Verification items for the finished model (mm, model axes). Face numbers are marked on the shaded views. A direction names the side the tool comes from. Round coordinates to 2 decimals unless told otherwise and drop trailing zeros. Write each loop counter-clockwise with the first axis right and the second up, starting at its lowest first coordinate (ties: lowest second). Pieces come first, ordered by that corner, then holes. Notation, with made-up numbers: M -37.5,61 L 3.5,61 A36 cw 3.5,97 Z; hole C 73.5,50 d11. An arc over 180 degrees is marked long. One line per item, written item: value. Start each with the question number.
Item 1: Section check D-D, the plane z = -10. Record the cut outline in (x, y), then the cut area to 3 significant figures.
Item 2: Gauge pin test, flat ends, axial feed: pin 1 (5.5 mm diameter, centred on x = 26, y = 11.5, fed in from +Z); pin 2 (12 mm diameter, centred on x = -13, y = 17, fed in from -Z); pin 3 (4 mm diameter, centred on x = 55.97, z = 20.76, fed in from +Y); pin 4 (3 mm diameter, centred on y = 13.5, z = 16, fed in from -X). Record the tip position at first contact, or that the pin passes through.
Item 3: Thickness scan on probe 1 along X at (y, z) = (31.5, -2); probe 2 along Y at (x, z) = (48.5, -8); probe 3 along Y at (x, z) = (-3, -3). Record the ranges inside material, lowest first. Write a range as from..to.
Item 4: Tool access check on the marked faces 5, 6, 7 and 8. Record the directions out of +Z, -Z, +X, -X, +Y, -Y that give a thin tool (end or side, any length) a straight path to the whole face; none if there is none.
Item 5: Draft check along X on the marked faces 1, 2, 3 and 4. Enter one of: +X half, -X half, draft (parallel to the pull), parting line (faces both ways), or undercut.
Item 6: Section check B-B, the plane y = 7. Record the cut outline in (x, z).
Item 7: Section check A-A, the plane y = 12.5. Record the cut outline in (x, z), then the cut area to 3 significant figures.
Item 8: Section check C-C, the plane x = 39.5. Record the cut outline in (y, z).
from build123d import *

# Parameters (mm, degrees)
CROQUIS1_W              = 98
CROQUIS1_H              = 53
SALIENTE_EXTRUIR1_DEPTH = 35
CROQUIS2_R              = 1.052356083
CORTAR_EXTRUIR1_DEPTH   = 25
CROQUIS4_R              = 1.21
CORTAR_EXTRUIR2_DEPTH   = 77.456439381
CROQUIS5_R              = 1.21
CORTAR_EXTRUIR3_DEPTH   = 77.456439381
CROQUIS6_W              = 19.087146806
CROQUIS6_H              = 12.5
CORTAR_EXTRUIR4_DEPTH   = 99.715019882
CROQUIS7_W              = 19.109936399
CROQUIS7_H              = 12.5
CORTAR_EXTRUIR5_DEPTH   = 95.352926478
CORTAR_EXTRUIR6_DEPTH   = 83.575081806
CORTAR_EXTRUIR7_DEPTH   = 30
CORTAR_EXTRUIR8_DEPTH   = 110.416374403
CORTAR_EXTRUIR9_DEPTH   = 24
CROQUIS12_W             = 107.668440241
CROQUIS12_H             = 57.968086936
CORTAR_EXTRUIR10_DEPTH  = 2.5
CORTAR_EXTRUIR11_DEPTH  = 109.642500834


with BuildPart() as part:
    # Croquis1 → Saliente-Extruir1 (new body)
    with BuildSketch(Plane(origin=(0, 0, 0), x_dir=(1, 0, 0), z_dir=(0, 1, 0))):
        with Locations((9.971553611, -7.307439825)):
            Rectangle(CROQUIS1_W, CROQUIS1_H)
    extrude(amount=SALIENTE_EXTRUIR1_DEPTH)

    # Croquis2 → Cortar-Extruir1 (cut)
    with BuildSketch(Plane(origin=(0, 35, 0), x_dir=(1, 0, 0), z_dir=(0, 1, 0))):
        Polygon((19.971553611, -26.807439825), (9.971553611, -26.807439825), (-0.028446389, -26.807439825), (-21.028702453, -26.807439825), (-36.028446389, -15.003760101), (-39.028446389, -12.284028263), (-39.028446389, -33.807439825), (58.971553611, -33.807439825), (58.971553611, -10.155599963), (55.971553611, -15.003760101), (40.942820659, -26.807439825), align=None)
        with Locations(Location((-36.028446389, -20.755083742, 0), (0, 0, 270))):
            Circle(CROQUIS2_R, mode=Mode.SUBTRACT)
        with Locations(Location((55.971553611, -20.755083742, 0), (0, 0, 270))):
            Circle(CROQUIS2_R, mode=Mode.SUBTRACT)
    extrude(amount=-CORTAR_EXTRUIR1_DEPTH, mode=Mode.SUBTRACT)

    # Croquis4 → Cortar-Extruir2 (cut, through all)
    with BuildSketch(Plane(origin=(0, 35, 0), x_dir=(1, 0, 0), z_dir=(0, 1, 0))):
        with Locations(Location((-36.028446389, -20.755083742, 0), (0, 0, 270))):
            Circle(CROQUIS4_R)
    extrude(amount=-CORTAR_EXTRUIR2_DEPTH, mode=Mode.SUBTRACT)

    # Croquis5 → Cortar-Extruir3 (cut, through all)
    with BuildSketch(Plane(origin=(0, 35, 0), x_dir=(1, 0, 0), z_dir=(0, 1, 0))):
        with Locations(Location((55.971553611, -20.755083742, 0), (0, 0, 270))):
            Circle(CROQUIS5_R)
    extrude(amount=-CORTAR_EXTRUIR3_DEPTH, mode=Mode.SUBTRACT)

    # Croquis6 → Cortar-Extruir4 (cut, through all)
    with BuildSketch(Plane(origin=(-21.069927214, 0, 26.774999013), x_dir=(0.7858557430790737, 0, 0.6184098568664935), z_dir=(-0.6184098568664935, 0, 0.7858557430790737))):
        with Locations((-9.49111497, 16.25)):
            Rectangle(CROQUIS6_W, CROQUIS6_H)
    extrude(amount=-CORTAR_EXTRUIR4_DEPTH, mode=Mode.SUBTRACT)

    # Croquis7 → Cortar-Extruir5 (cut, through all)
    with BuildSketch(Plane(origin=(28.642438973, 0, 36.468251975), x_dir=(0.7864355295732114, 0, -0.6176723709418307), z_dir=(0.6176723709418307, 0, 0.7864355295732114))):
        with Locations((25.195642131, 16.25)):
            Rectangle(CROQUIS7_W, CROQUIS7_H)
    extrude(amount=-CORTAR_EXTRUIR5_DEPTH, mode=Mode.SUBTRACT)

    # Croquis8 → Cortar-Extruir6 (cut, through all)
    with BuildSketch(Plane.XY.offset(26.807439825)):
        Polygon((9.971553611, 10), (0.071553611, 10), (0.071553611, 22.5), (9.971553611, 22.5), (19.871553611, 22.5), (19.871553611, 10), align=None)
    extrude(amount=-CORTAR_EXTRUIR6_DEPTH, mode=Mode.SUBTRACT)

    # Croquis9 → Cortar-Extruir7 (cut)
    with BuildSketch(Plane(origin=(0, 35, 0), x_dir=(1, 0, 0), z_dir=(0, 1, 0))):
        Polygon((9.971553611, 15.192560175), (42.971553611, 15.192560175), (42.971553611, -5.347439825), (9.971553611, -5.347439825), (-23.028446389, -5.347439825), (-23.028446389, 15.192560175), align=None)
    extrude(amount=-CORTAR_EXTRUIR7_DEPTH, mode=Mode.SUBTRACT)

    # Croquis10 → Cortar-Extruir8 (cut, through all)
    with BuildSketch(Plane(origin=(58.971553611, 0, 0), x_dir=(0, 0, -1), z_dir=(1, 0, 0))):
        Polygon((4.518480106, 10), (11.018480106, 10), (11.018480106, 30.02), (4.518480106, 30.02), (-1.981519894, 30.02), (-1.981519894, 10), align=None)
    extrude(amount=-CORTAR_EXTRUIR8_DEPTH, mode=Mode.SUBTRACT)

    # Croquis11 → Cortar-Extruir9 (cut)
    with BuildSketch(Plane(origin=(0, 0, -19.192560175), x_dir=(-1, 0, 0), z_dir=(0, 0, -1))):
        Polygon((-9.971553611, 35), (23.028446389, 35), (23.028446389, 10), (-9.971553611, 10), (-42.971553611, 10), (-42.971553611, 35), align=None)
    extrude(amount=-CORTAR_EXTRUIR9_DEPTH, mode=Mode.SUBTRACT)

    # Croquis12 → Cortar-Extruir10 (cut)
    with BuildSketch(Plane(origin=(0, 35, 0), x_dir=(1, 0, 0), z_dir=(0, 1, 0))):
        with Locations((11.756632462, -7.871148936)):
            Rectangle(CROQUIS12_W, CROQUIS12_H)
    extrude(amount=-CORTAR_EXTRUIR10_DEPTH, mode=Mode.SUBTRACT)

    # Croquis13 → Cortar-Extruir11 (cut, through all)
    with BuildSketch(Plane(origin=(58.971553611, 0, 0), x_dir=(0, 0, -1), z_dir=(1, 0, 0))):
        Polygon((-33.807439825, 32.5), (-33.807439825, 10), (-31.442255839, 10), (-10.155599963, 32.5), align=None)
    extrude(amount=-CORTAR_EXTRUIR11_DEPTH, mode=Mode.SUBTRACT)


solid = part.part
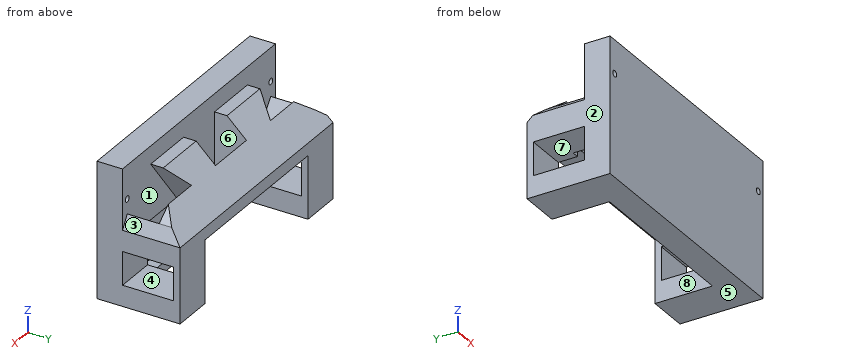
Response values:
1. outline: M -39.03,0 L 58.97,0 L 58.97,10 L 42.97,10 L 42.97,5 L -23.03,5 L -23.03,10 L -39.03,10 Z; M -39.03,30.02 L -23.03,30.02 L -23.03,32.5 L -39.03,32.5 Z; M 42.97,30.02 L 58.97,30.02 L 58.97,32.5 L 42.97,32.5 Z
1. area: 729 mm2
2. pin 1: stops at z = 33.81
2. pin 2: stops at z = 5.35
2. pin 3: stops at y = 10
2. pin 4: stops at x = -36.58
3. probe 1: x = -39.03..-23.03, 42.97..58.97
3. probe 2: y = 0..10, 30.02..32.5
3. probe 3: y = 0..5
4. face 5: -Z, +X, -X, +Y, -Y
4. face 6: +Z, -Z
4. face 7: +X, -X
4. face 8: +Y
5. face 1: undercut
5. face 2: -X half
5. face 3: +X half
5. face 4: draft
6. outline: M -39.03,-19.19 L 58.97,-19.19 L 58.97,33.81 L -39.03,33.81 Z; hole C -36.03,20.76 d2.42; hole M -23.03,-15.19 L 42.97,-15.19 L 42.97,5.35 L -23.03,5.35 Z; hole C 55.97,20.76 d2.42
7. outline: M -39.03,-19.19 L -23.03,-19.19 L -23.03,-11.02 L -39.03,-11.02 Z; M -39.03,1.98 L -25.78,1.98 L -36.03,15 L -39.03,12.28 Z; M -21.03,26.81 L -4.14,5.35 L 0.07,5.35 L 0.07,26.81 Z; M 19.87,5.35 L 24.09,5.35 L 40.94,26.81 L 19.87,26.81 Z; M 42.97,-19.19 L 58.97,-19.19 L 58.97,-11.02 L 42.97,-11.02 Z; M 45.74,1.98 L 58.97,1.98 L 58.97,10.16 L 55.97,15 Z
7. area: 1,000 mm2
8. outline: M 0,-19.19 L 10,-19.19 L 10,-15.19 L 5,-15.19 L 5,5.35 L 10,5.35 L 10,24.97 L 16.84,24.97 L 14.9,26.81 L 10,26.81 L 10,33.81 L 0,33.81 Z; M 22.5,5.35 L 32.5,5.35 L 32.5,10.16 L 22.5,19.62 Z
